The model under review builds one solid part; all positions refer to its coordinate system, in mm. A direction names the side the tool comes from. Round coordinates to 2 decimals unless told otherwise and drop trailing zeros. Order: outer loops, then holes, each group sorted by start corner. A loop starts at its lowest first (then second) coordinate and runs counter-clockwise, first axis right, second up. Notation, with made-up numbers: (19, 65) -> (62, 65) arc R22 ccw to (62, 87) -> close; hole circle Ø3 at (53.5, 20.5). An arc over 180 degrees is marked (long way). Use a Markdown table: item, result. Add a question column.
```python
from build123d import *

# Parameters (mm, degrees)
EXTRUDE_1_DEPTH             = 103.907768917
SHELL_1_T                   = 3
HOLE_WIZARD_M3_1_D          = 3.4
SKETCH_6_W                  = 3
SKETCH_6_H                  = 95.907768917
EXTRUDE_2_DEPTH             = 10
SKETCH_10_R                 = 3
SKETCH_10_W                 = 10
SKETCH_10_H                 = 35.3
EXTRUDE_3_DEPTH             = 3
HOLE_WIZARD_M2_2_D          = 1.5
HOLE_WIZARD_M2_3_D          = 1.5
SKETCH_17_R                 = 1.8
SKETCH_17_R_2               = 0.75
SKETCH_17_W                 = 7.6
SKETCH_17_H                 = 10.2
CUT_EXTRUDE_1_DEPTH         = 3
FILLET_1_R                  = 1
TAP_DRILL_FOR_M2_TAP1_D     = 1.5
TAP_DRILL_FOR_M2_TAP1_DEPTH = 3


with BuildPart() as part:
    # 草图1 → 凸台-拉伸1 (new body)
    with BuildSketch(Plane.XY):
        with BuildLine():
            Line((113.912965174, -22.401534746), (113.912965174, -6.401534746))
            ThreePointArc((113.912965174, -6.401534746), (111.130479595, 0.315979676), (104.412965174, 3.098465254))
            Line((104.412965174, 3.098465254), (98.673756893, 3.098465254))
            Line((98.673756893, 3.098465254), (85.173756893, -10.401534746))
            Line((85.173756893, -10.401534746), (-26.759170781, -10.401534746))
            Line((-26.759170781, -10.401534746), (-26.759170781, -22.401534746))
            Line((-26.759170781, -22.401534746), (113.912965174, -22.401534746))
        make_face()
    extrude(amount=-EXTRUDE_1_DEPTH)

    # 抽壳1
    shell_1_openings = [part.faces().sort_by_distance(p)[0] for p in [
        (113.912965174, -14.401534746, -51.953884458),
        (111.130479595, 0.315979676, -51.953884458),
        (101.543361033, 3.098465254, -51.953884458),
        (91.923756893, -3.651534746, -51.953884458),
        (29.207293056, -10.401534746, -51.953884458),
    ]]
    offset(amount=SHELL_1_T, openings=shell_1_openings, kind=Kind.INTERSECTION)

    # M3 间隙孔1 (through all)
    with Locations(Plane.XY.offset(3)):
        with Locations((104.412965174, -6.401534746)):
            Hole(HOLE_WIZARD_M3_1_D / 2)

    # 草图6 → 凸台-拉伸2 (add)
    with BuildSketch(Plane(origin=(0, -22.401534746, 0), x_dir=(1, 0, 0), z_dir=(0, 1, 0))):
        with Locations((98.543945955, 51.453884459)):
            Rectangle(SKETCH_6_W, SKETCH_6_H)
    extrude(amount=EXTRUDE_2_DEPTH)

    # 草图10 → 凸台-拉伸3 (add)
    with BuildSketch(Plane(origin=(0, -22.401534746, 0), x_dir=(1, 0, 0), z_dir=(0, 1, 0))):
        with Locations((67.811261753, 78.757768917)):
            Circle(SKETCH_10_R)
        with Locations((67.811261753, 43.457768917)):
            Circle(SKETCH_10_R)
        with Locations((67.811261753, 61.107768917)):
            Rectangle(SKETCH_10_W, SKETCH_10_H)
        with BuildLine():
            ThreePointArc((64.811261753, 43.457768917), (67.811261753, 40.457768917), (70.811261753, 43.457768917))
            Line((70.811261753, 43.457768917), (64.811261753, 43.457768917))
        make_face()
        with BuildLine():
            Line((64.811261753, 43.457768917), (70.811261753, 43.457768917))
            ThreePointArc((70.811261753, 43.457768917), (67.811261753, 46.457768917), (64.811261753, 43.457768917))
        make_face()
        with BuildLine():
            ThreePointArc((64.811261753, 78.757768917), (67.811261753, 75.757768917), (70.811261753, 78.757768917))
            Line((70.811261753, 78.757768917), (64.811261753, 78.757768917))
        make_face()
        with BuildLine():
            Line((64.811261753, 78.757768917), (70.811261753, 78.757768917))
            ThreePointArc((70.811261753, 78.757768917), (67.811261753, 81.757768917), (64.811261753, 78.757768917))
        make_face()
    extrude(amount=EXTRUDE_3_DEPTH)

    # M2 螺纹孔的螺纹孔钻头2 (through all)
    with Locations(Plane(origin=(0, -19.401534746, 0), x_dir=(1, 0, 0), z_dir=(0, 1, 0))):
        with Locations((67.811261753, 43.457768917), (67.811261753, 78.757768917)):
            Hole(HOLE_WIZARD_M2_2_D / 2)

    # M2 螺纹孔的螺纹孔钻头3 (through all)
    with Locations(Plane(origin=(0, -22.401534746, 0), x_dir=(1, 0, 0), z_dir=(0, 1, 0))):
        with Locations((19.856566152, 43.457768917), (19.856566152, 78.757768917)):
            Hole(HOLE_WIZARD_M2_3_D / 2)

    # 草图17 → 切除-拉伸1 (cut)
    with BuildSketch(Plane.XZ.offset(25.401534746)):
        with Locations((56.1974918, -15.765719737)):
            Circle(SKETCH_17_R)
        with Locations((81.7174918, -23.765719737)):
            Circle(SKETCH_17_R_2)
        with Locations((76.5474918, -16.415719737)):
            Rectangle(SKETCH_17_W, SKETCH_17_H)
    extrude(amount=-CUT_EXTRUDE_1_DEPTH, mode=Mode.SUBTRACT)

    # 圆角1
    fillet_1_edges = [part.edges().sort_by_distance(p)[0] for p in [
        (100.043945955, -22.401534746, -51.453884458),
    ]]
    fillet(fillet_1_edges, radius=FILLET_1_R)

    # Tap Drill for M2 Tap1
    with Locations(Plane.ZY.offset(29.759170781)):
        with Locations((-2.818814719, -20.846782883), (-1.181185281, -14.956286608), (-102.726583636, -20.846782883), (-101.088954197, -14.956286608)):
            Hole(TAP_DRILL_FOR_M2_TAP1_D / 2, depth=TAP_DRILL_FOR_M2_TAP1_DEPTH)


solid = part.part
```
Q1. For faces 1 (the face through (76, -24, -21.516)), 2 (the face through (100.044, -17, -51)), 3 (the face through (62.811, -21, -61)), list the 3-axis set-ups (+Z, -Z, +X, -X, +Y, -Y) from which the entire face can be reached by the end or side of a thin tool; tool diameter is ignored.
Q2. Draft analysis for pull direction Y (two halves, no side actions). For faces 4 (the face through (106.11, -6.33, 1.48)), 5 (the face through (67.877, -20.923, -81.757)), 6 (the face through (111.204, 0.242, 1.521)), state which applies: released by +Y, released by -Y, zero draft, split by the parting line, or undercut.
Q3. To check wall thickness, follow line 1 along Z through (x, y) = (55, -16.75); line 2 along X through (y, z) = (-19.5, -38.5); line 3 along Z through (x, y) = (69, -19.5). State the ranges of each line that lie inside material, in increasing order.
Q4. Add section B-B, the plane x = -2. Give the boundary of the cut face in (y, z).
Q5. Add section A-A, the plane y = -2.5. Give the boundary of the cut face in (x, z), then the cut area to 3 significant figures.
Q6. Add section D-D, the plane z = -92.5. Give the boundary of the cut face in (x, y), then the cut area to 3 significant figures.
Q7. Add section C-C, the plane z = -46. Give the boundary of the cut face in (x, y), then the cut area to 3 significant figures.
Q8. For pin 1 (2 mm diameter, centred on x = 12.5, z = -74, fed in from +Y), flat-tipped, find the tip position at first contact; note if it passes through.
Return value:
| question | item | result |
|---|---|---|
| 1 | face 1 | +Y, -Y |
| 1 | face 2 | +X, +Y |
| 1 | face 3 | +Y |
| 2 | face 4 | undercut |
| 2 | face 5 | zero draft |
| 2 | face 6 | released by +Y |
| 3 | line 1 | -106.91 to -103.91, 0 to 3 |
| 3 | line 2 | -29.76 to -26.76, 97.04 to 100.04 |
| 3 | line 3 | -106.91 to -103.91, -81.51 to -40.7, 0 to 3 |
| 4 | outline | (-25.4, -106.91) -> (-10.4, -106.91) -> (-10.4, -103.91) -> (-22.4, -103.91) -> (-22.4, 0) -> (-10.4, 0) -> (-10.4, 3) -> (-25.4, 3) -> close |
| 5 | outline | (93.08, -106.91) -> (113.07, -106.91) -> (113.07, -103.91) -> (93.08, -103.91) -> close; (93.08, 0) -> (113.07, 0) -> (113.07, 3) -> (93.08, 3) -> close |
| 5 | area | 120 mm² |
| 6 | outline | (-29.76, -25.4) -> (113.91, -25.4) -> (113.91, -22.4) -> (101.04, -22.4) arc R1 cw to (100.04, -21.4) -> (100.04, -12.4) -> (97.04, -12.4) -> (97.04, -22.4) -> (-26.76, -22.4) -> (-26.76, -10.4) -> (-29.76, -10.4) -> close |
| 6 | area | 497 mm² |
| 7 | outline | (-29.76, -25.4) -> (113.91, -25.4) -> (113.91, -22.4) -> (101.04, -22.4) arc R1 cw to (100.04, -21.4) -> (100.04, -12.4) -> (97.04, -12.4) -> (97.04, -22.4) -> (72.81, -22.4) -> (72.81, -19.4) -> (62.81, -19.4) -> (62.81, -22.4) -> (-26.76, -22.4) -> (-26.76, -10.4) -> (-29.76, -10.4) -> close |
| 7 | area | 527 mm² |
| 8 | pin 1 | y = -22.4 |
